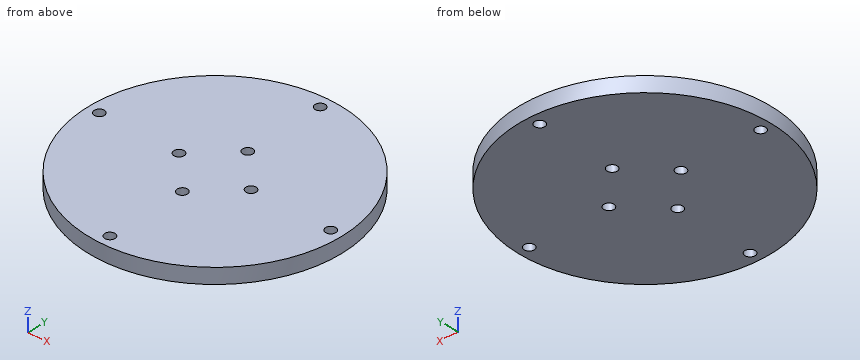
```python
from build123d import *

# Parameters (mm, degrees)
SKETCH1_R           = 25
SKETCH1_R_2         = 1
BOSS_EXTRUDE1_DEPTH = 1.5


with BuildPart() as part:
    # Sketch1 → Boss-Extrude1 (new, symmetric)
    with BuildSketch(Plane.XY):
        Circle(SKETCH1_R)
        with Locations((0, 22.715)):
            Circle(SKETCH1_R_2, mode=Mode.SUBTRACT)
        with Locations((0, 7.071067812)):
            Circle(SKETCH1_R_2, mode=Mode.SUBTRACT)
        with Locations((7.071067812, 0)):
            Circle(SKETCH1_R_2, mode=Mode.SUBTRACT)
        with Locations((0, -7.071067812)):
            Circle(SKETCH1_R_2, mode=Mode.SUBTRACT)
        with Locations((-7.071067812, 0)):
            Circle(SKETCH1_R_2, mode=Mode.SUBTRACT)
        with Locations((22.715, 0)):
            Circle(SKETCH1_R_2, mode=Mode.SUBTRACT)
        with Locations((0, -22.715)):
            Circle(SKETCH1_R_2, mode=Mode.SUBTRACT)
        with Locations((-22.715, 0)):
            Circle(SKETCH1_R_2, mode=Mode.SUBTRACT)
    extrude(amount=BOSS_EXTRUDE1_DEPTH, both=True)


solid = part.part
```
Input: part model. Units: mm. Frame: model coordinates. Give positions to 0.01 mm unless a question says otherwise; leave off trailing zeros. Order: outer loops, then holes, each group sorted by start corner. A loop starts at its lowest first (then second) coordinate and runs counter-clockwise, first axis right, second up. Notation, with made-up numbers: (60, 70) - (102, 70) arc R8 cw to (102, 84) - close; hole circle Ø4 at (65, 70). An arc over 180 degrees is marked (long way). Use a Markdown table: item, result.
(1) Line query: line 1 (Y direction, x = 0, z = 0.3) (3 decimals); line 2 (X direction, y = 0.5, z = -1.3) (3 decimals); line 3 (X direction, y = -6.5, z = 0.3). Output: solid intervals per line, ascending. Write a range as from..to.
Computed values:
| item | result |
|---|---|
| line 1 | y = -25..-23.715, -21.715..-8.071, -6.071..6.071, 8.071..21.715, 23.715..25 |
| line 2 | x = -24.995..-23.581, -21.849..-7.937, -6.205..6.205, 7.937..21.849, 23.581..24.995 |
| line 3 | x = -24.14..-0.82, 0.82..24.14 |
(2) Pin query (flat end, axial travel): pin 1 (2.5 mm diameter, centred on x = 0, y = 22.715, fed in from +Z); pin 2 (1 mm diameter, centred on x = -3, z = 0.5, fed in from +Y). Return the tip coordinate at first contact, or that it passes through.
Computed values:
| item | result |
|---|---|
| pin 1 | stops at z = 1.5 |
| pin 2 | stops at y = 24.87 |
(3) Section query A-A (x = 0). Output: boundary loops of the cut face in (y, z) (3 decimals), then the cut area to 3 significant figures.
Computed values:
| item | result |
|---|---|
| outline | (-25, -1.5) - (-23.715, -1.5) - (-23.715, 1.5) - (-25, 1.5) - close; (-21.715, -1.5) - (-8.071, -1.5) - (-8.071, 1.5) - (-21.715, 1.5) - close; (-6.071, -1.5) - (6.071, -1.5) - (6.071, 1.5) - (-6.071, 1.5) - close; (8.071, -1.5) - (21.715, -1.5) - (21.715, 1.5) - (8.071, 1.5) - close; (23.715, -1.5) - (25, -1.5) - (25, 1.5) - (23.715, 1.5) - close |
| area | 126 mm2 |
(4) Section query C-C (z = 0.9). State how many separate pieces and enclosed holes the cut face has, then the cut area to 3 significant figures.
Computed values:
| item | result |
|---|---|
| separate pieces | 1 |
| enclosed holes | 8 |
| area | 1,940 mm2 |
(5) Section query D-D (y = 20). Output: boundary loops of the cut face in (x, z), then the cut area to 3 significant figures.
Computed values:
| item | result |
|---|---|
| outline | (-15, -1.5) - (15, -1.5) - (15, 1.5) - (-15, 1.5) - close |
| area | 90.0 mm2 |
